```python
from build123d import *

# Parameters (mm, degrees)
SKETCH_1_W          = 80
SKETCH_1_H          = 32
EXTRUDE_1_DEPTH     = 50
HOLE_WIZARD_M16_1_D = 14
SKETCH_5_R          = 5
CUT_EXTRUDE_1_DEPTH = 67


with BuildPart() as part:
    # 草图1 → 凸台-拉伸1 (new body)
    with BuildSketch(Plane(origin=(0, 0, 0), x_dir=(0, 0, -1), z_dir=(1, 0, 0))):
        Rectangle(SKETCH_1_W, SKETCH_1_H)
    extrude(amount=EXTRUDE_1_DEPTH)

    # M16 螺纹孔1 (through all)
    with Locations(Plane.ZY):
        with Locations((0, 0)):
            Hole(HOLE_WIZARD_M16_1_D / 2)

    # 草图5 → 切除-拉伸1 (cut, through all)
    with BuildSketch(Plane.ZY):
        with Locations((30, 0)):
            Circle(SKETCH_5_R)
    cut_extrude_1 = extrude(amount=-CUT_EXTRUDE_1_DEPTH, mode=Mode.SUBTRACT)

    # 镜向1: 切除-拉伸1 across plane
    add(cut_extrude_1.mirror(Plane.XY), mode=Mode.SUBTRACT)


solid = part.part
```
For this review, take the finished solid that the model builds, in its own axes (mm). Give positions to 0.01 mm unless a question says otherwise; leave off trailing zeros. Order: outer loops, then holes, each group sorted by start corner. A loop starts at its lowest first (then second) coordinate and runs counter-clockwise, first axis right, second up.
1) The part is to be moulded in two halves that separate along Y. For faces 1 (the face through (25, 0, 25)), 2 (the face through (25, -16, 1)), 3 (the face through (25, 16, 1)), say which applies: released by +Y, released by -Y, zero draft, split by the parting line, or undercut.
2) Take a section at C-C (y = 0). Give the boundary of the cut face in (x, z).
3) Take a section at A-A (z = 30). Give the boundary of the cut face in (x, y).
4) Take a section at B-B (x = 24). Give the boundary of the cut face in (y, z).
5) Wall thickness on line 1 (Y direction, x = 31.5, z = 0); line 2 (Y direction, x = 15, z = -30): over which ranges is each line inside the solid? List them lowest first.
6) Insertion check: pin 1 (9 mm diameter, centred on y = 0, z = -30, fed in from +X). The pin has a flat end and moves straight along its axis. Give the tip position at first contact, or say it passes through.
Derived:
1. face 1: undercut
1. face 2: released by -Y
1. face 3: released by +Y
2. outline: (0, -40) - (50, -40) - (50, -35) - (0, -35) - close; (0, -25) - (50, -25) - (50, -7) - (0, -7) - close; (0, 7) - (50, 7) - (50, 25) - (0, 25) - close; (0, 35) - (50, 35) - (50, 40) - (0, 40) - close
3. outline: (0, -16) - (50, -16) - (50, -5) - (0, -5) - close; (0, 5) - (50, 5) - (50, 16) - (0, 16) - close
4. outline: (-16, -40) - (16, -40) - (16, 40) - (-16, 40) - close; hole circle Ø14 at (0, 0); hole circle Ø10 at (0, -30); hole circle Ø10 at (0, 30)
5. line 1: y = -16 to -7, 7 to 16
5. line 2: y = -16 to -5, 5 to 16
6. pin 1: passes through
